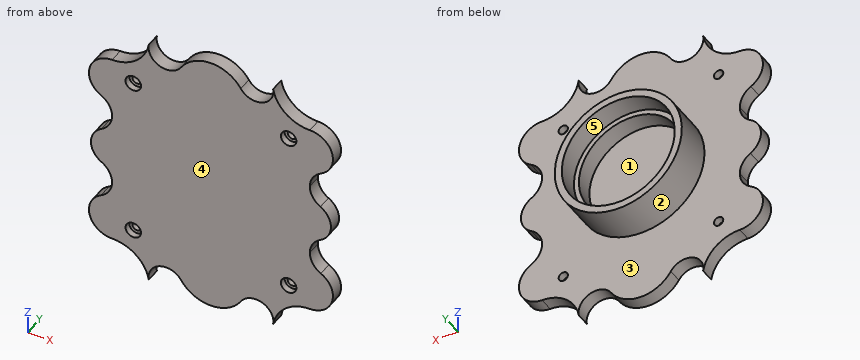
from build123d import *

# Parameters (mm, degrees)
SALIENTE_EXTRUIR1_DEPTH                              = 10
SALIENTE_EXTRUIR2_DEPTH                              = 10
CROQUIS3_R                                           = 40
CROQUIS3_R_2                                         = 36.5
SALIENTE_EXTRUIR3_DEPTH                              = 13
CROQUIS4_R                                           = 45
CROQUIS4_R_2                                         = 40
SALIENTE_EXTRUIR4_DEPTH                              = 28
REFRENTADO_PARA_TORNILLO_CON_CABEZA_HUEC_D           = 6.6
REFRENTADO_PARA_TORNILLO_CON_CABEZA_HUEC_CBORE_D     = 11
REFRENTADO_PARA_TORNILLO_CON_CABEZA_HUEC_CBORE_DEPTH = 4.6


with BuildPart() as part:
    # Croquis1 → Saliente-Extruir1 (new body)
    with BuildSketch(Plane(origin=(0, 0, 0), x_dir=(1, 0, 0), z_dir=(0, 1, 0))):
        with BuildLine():
            Line((-70, -70), (-70, 70))
            ThreePointArc((-70, 70), (-52.983030462, 76.249658661), (-44.055908755, 92.027554074))
            ThreePointArc((-44.055908755, 92.027554074), (-36.156795126, 78.313355526), (-21.147629234, 83.333333333))
            ThreePointArc((-21.147629234, 83.333333333), (0, 95), (21.147629234, 83.333333333))
            ThreePointArc((21.147629234, 83.333333333), (36.156795126, 78.313355526), (44.055908755, 92.027554074))
            ThreePointArc((44.055908755, 92.027554074), (52.983030462, 76.249658661), (70, 70))
            Line((70, 70), (70, -70))
            ThreePointArc((70, -70), (52.983030462, -76.249658661), (44.055908755, -92.027554074))
            ThreePointArc((44.055908755, -92.027554074), (36.156795126, -78.313355526), (21.147629234, -83.333333333))
            ThreePointArc((21.147629234, -83.333333333), (0, -95), (-21.147629234, -83.333333333))
            ThreePointArc((-21.147629234, -83.333333333), (-36.156795126, -78.313355526), (-44.055908755, -92.027554074))
            ThreePointArc((-44.055908755, -92.027554074), (-52.983030462, -76.249658661), (-70, -70))
        make_face()
    extrude(amount=SALIENTE_EXTRUIR1_DEPTH)

    # Croquis2 → Saliente-Extruir2 (add)
    with BuildSketch(Plane(origin=(0, 10, 0), x_dir=(1, 0, 0), z_dir=(0, 1, 0))):
        with BuildLine():
            Line((-70, 25.98076189), (-70, 70))
            ThreePointArc((-70, 70), (-85.909969357, 57.627811916), (-77.837993487, 39.160506523))
            ThreePointArc((-77.837993487, 39.160506523), (-72.107558403, 33.647896498), (-70, 25.98076189))
        make_face()
        with BuildLine():
            ThreePointArc((77.837993487, 39.160506523), (85.909969357, 57.627811916), (70, 70))
            Line((70, 70), (70, 25.98076213))
            ThreePointArc((70, 25.98076213), (72.107558465, 33.647896602), (77.837993487, 39.160506523))
        make_face()
        with BuildLine():
            ThreePointArc((77.5, 12.990381057), (72.009618939, 18.480762121), (70, 25.98076213))
            Line((70, 25.98076213), (70, -25.98076213))
            ThreePointArc((70, -25.98076213), (72.009618939, -18.480762121), (77.5, -12.990381057))
            ThreePointArc((77.5, -12.990381057), (85, 0), (77.5, 12.990381057))
        make_face()
        with BuildLine():
            Line((-70, -25.980762199), (-70, 25.98076189))
            ThreePointArc((-70, 25.98076189), (-72.009618999, 18.480762017), (-77.5, 12.990381057))
            ThreePointArc((-77.5, 12.990381057), (-85, 0), (-77.5, -12.990381057))
            ThreePointArc((-77.5, -12.990381057), (-72.009618922, -18.480762151), (-70, -25.980762199))
        make_face()
        with BuildLine():
            Line((-70, -70), (-70, -25.980762199))
            ThreePointArc((-70, -25.980762199), (-72.107558482, -33.647896631), (-77.837993487, -39.160506523))
            ThreePointArc((-77.837993487, -39.160506523), (-85.909969357, -57.627811916), (-70, -70))
        make_face()
        with BuildLine():
            ThreePointArc((77.837993487, -39.160506523), (72.107558465, -33.647896602), (70, -25.98076213))
            Line((70, -25.98076213), (70, -70))
            ThreePointArc((70, -70), (85.909969357, -57.627811916), (77.837993487, -39.160506523))
        make_face()
    extrude(amount=-SALIENTE_EXTRUIR2_DEPTH)

    # Croquis3 → Saliente-Extruir3 (add)
    with BuildSketch(Plane(origin=(0, 10, 0), x_dir=(1, 0, 0), z_dir=(0, 1, 0))):
        with Locations(Location((0, 0, 0), (0, 0, 90))):
            Circle(CROQUIS3_R)
        with Locations(Location((0, 0, 0), (0, 0, 90))):
            Circle(CROQUIS3_R_2, mode=Mode.SUBTRACT)
    extrude(amount=SALIENTE_EXTRUIR3_DEPTH)

    # Croquis4 → Saliente-Extruir4 (add)
    with BuildSketch(Plane(origin=(0, 10, 0), x_dir=(1, 0, 0), z_dir=(0, 1, 0))):
        with Locations(Location((0, 0, 0), (0, 0, 270))):
            Circle(CROQUIS4_R)
        with Locations(Location((0, 0, 0), (0, 0, 270))):
            Circle(CROQUIS4_R_2, mode=Mode.SUBTRACT)
    extrude(amount=SALIENTE_EXTRUIR4_DEPTH)

    # Refrentado para tornillo con cabeza hueca hexagonal de M61 (through all)
    with Locations(Plane(origin=(-55, 0, 57.5), x_dir=(0, 0, -1), z_dir=(0, -1, 0))):
        with Locations((0, 0), (0, 110), (115, 110), (115, 0)):
            CounterBoreHole(REFRENTADO_PARA_TORNILLO_CON_CABEZA_HUEC_D / 2, REFRENTADO_PARA_TORNILLO_CON_CABEZA_HUEC_CBORE_D / 2, REFRENTADO_PARA_TORNILLO_CON_CABEZA_HUEC_CBORE_DEPTH)


solid = part.part
Geometry check sheet. Reference: the model listing, model coordinates, mm. Face numbers are marked on the shaded views. A direction names the side the tool comes from. Give positions to 0.01 mm unless a question says otherwise; leave off trailing zeros. Order: outer loops, then holes, each group sorted by start corner. A loop starts at its lowest first (then second) coordinate and runs counter-clockwise, first axis right, second up.
1. Draft check along Z on the marked faces 1, 2 and 3. Enter one of: pulls with the +Z half, pulls with the -Z half, needs draft (parallel to the pull), parting line crosses it, or undercut.
Completed:
face 1: undercut
face 2: parting line crosses it
face 3: needs draft
2. Access from +Z, -Z, +X, -X, +Y, -Y to the whole of each face (thin tool, end or side, straight path). Record for the marked faces 4 and 5.
Completed:
face 4: +Z, -Z, +X, -X, -Y
face 5: +Y
3. Sectioned sample at B-B (z = 0). Record the boundary of the cut face in (x, y).
Completed:
outline: (-85, 0) - (85, 0) - (85, 10) - (45, 10) - (45, 38) - (40, 38) - (40, 23) - (36.5, 23) - (36.5, 10) - (-36.5, 10) - (-36.5, 23) - (-40, 23) - (-40, 38) - (-45, 38) - (-45, 10) - (-85, 10) - close
4. Sectioned sample at D-D (x = 0). Record the boundary of the cut face in (y, z).
Completed:
outline: (0, -95) - (10, -95) - (10, -45) - (38, -45) - (38, -40) - (23, -40) - (23, -36.5) - (10, -36.5) - (10, 36.5) - (23, 36.5) - (23, 40) - (38, 40) - (38, 45) - (10, 45) - (10, 95) - (0, 95) - close
5. Depth check by flat-ended pin: pin 1 (8.5 mm diameter, centred on x = -55, z = 57.5, fed in from +Y); pin 2 (9 mm diameter, centred on x = 55, z = 57.5, fed in from -Y); pin 3 (8 mm diameter, centred on x = 7, y = 17, fed in from +Z). Enter the tip coordinate at first touch or a pass-through.
Completed:
pin 1: stops at y = 10
pin 2: stops at y = 4.6
pin 3: stops at z = 44.9
6. Sectioned sample at A-A (z = 57.5). Record the boundary of the cut face in (x, y).
Completed:
outline: (-85.94, 0) - (-60.5, 0) - (-60.5, 4.6) - (-58.3, 4.6) - (-58.3, 10) - (-85.94, 10) - close; (-51.7, 4.6) - (-49.5, 4.6) - (-49.5, 0) - (49.5, 0) - (49.5, 4.6) - (51.7, 4.6) - (51.7, 10) - (-51.7, 10) - close; (58.3, 4.6) - (60.5, 4.6) - (60.5, 0) - (85.94, 0) - (85.94, 10) - (58.3, 10) - close
7. Scan lines: line 1 (X direction, y = 2, z = 57); line 2 (Y direction, x = 35, z = -70); line 3 (X direction, y = 4.5, z = 26). Record each from-to range of solid material in increasing order.
Completed:
line 1: x = -86.06 to -60.48, -49.52 to 49.52, 60.48 to 86.06
line 2: y = 0 to 10
line 3: x = -70 to 70
8. Sectioned sample at C-C (y = 18). Record the boundary of the cut face in (x, z), then the cut area to 3 significant figures.
Completed:
outline: circle Ø90 at (0, 0); hole circle Ø73 at (0, 0)
area: 2,180 mm2
